from build123d import *

# Parameters (mm, degrees)
F0_W      = 254
F0_H      = 203.2
F1_DEPTH  = 3.175
F3_DEPTH  = 25.4
F4_W      = 76.708
F4_H      = 76.708
F5_DEPTH  = 25.4
F6_R      = 38.354
F7_DEPTH  = 25.4
F9_DEPTH  = 25.4
F10_R     = 19.0754
F11_DEPTH = 25.4
F12_W     = 38.608
F12_H     = 38.608
F13_DEPTH = 25.4


with BuildPart() as f1:
    # F0 (on Top) → F1 (new body)
    with BuildSketch(Plane.XY):
        Rectangle(F0_W, F0_H)
    extrude(amount=F1_DEPTH)

    # F2 (on face) → F3 (cut)
    with BuildSketch(Plane(origin=(0, 0, 0), x_dir=(1, 0, 0), z_dir=(0, 0, -1))):
        Polygon((-69.596, 82.55), (-107.95, 5.842), (-31.242, 5.842), align=None)
    extrude(amount=-F3_DEPTH, mode=Mode.SUBTRACT)

    # F4 (on face) → F5 (cut)
    with BuildSketch(Plane(origin=(0, 0, 0), x_dir=(1, 0, 0), z_dir=(0, 0, -1))):
        with Locations((12.446, -44.196)):
            Rectangle(F4_W, F4_H)
    extrude(amount=-F5_DEPTH, mode=Mode.SUBTRACT)

    # F6 (on face) → F7 (cut)
    with BuildSketch(Plane(origin=(0, 0, 0), x_dir=(1, 0, 0), z_dir=(0, 0, -1))):
        with Locations((68.326, 45.466)):
            Circle(F6_R)
    extrude(amount=-F7_DEPTH, mode=Mode.SUBTRACT)

    # F8 (on face) → F9 (cut)
    with BuildSketch(Plane(origin=(0, 0, 0), x_dir=(1, 0, 0), z_dir=(0, 0, -1))):
        Polygon((94.512347, -42.973466), (75.208347, -81.581466), (113.816347, -81.581466), align=None)
    extrude(amount=-F9_DEPTH, mode=Mode.SUBTRACT)

    # F10 (on face) → F11 (cut)
    with BuildSketch(Plane(origin=(0, 0, 0), x_dir=(1, 0, 0), z_dir=(0, 0, -1))):
        with Locations((-76.1746, -44.4246)):
            Circle(F10_R)
    extrude(amount=-F11_DEPTH, mode=Mode.SUBTRACT)

    # F12 (on face) → F13 (cut)
    with BuildSketch(Plane(origin=(0, 0, 0), x_dir=(1, 0, 0), z_dir=(0, 0, -1))):
        with Locations((-10.528486, 59.436)):
            Rectangle(F12_W, F12_H)
    extrude(amount=-F13_DEPTH, mode=Mode.SUBTRACT)


solid = f1.part
Work out the finished part from the listing and answer in its coordinate system (mm). A direction names the side the tool comes from. Give positions to 0.01 mm unless a question says otherwise; leave off trailing zeros. Loops run counter-clockwise (first coordinate to the right, second up) from the corner with the lowest first, then second, coordinate; pieces in that order, holes last. Notation, with made-up numbers: (-39, 69) -> (-11, 69) arc R14 ccw to (-11, 83) -> close; hole circle Ø2 at (-38.75, 15.25). An arc over 180 degrees is marked (long way). Use a Markdown table: item, result. Add a question column.
1) For a pull along Y with two mould halves and no side action, classify faces 1 (the flat face through (-50.15, -43.66, 1.57)), 2 (the flat face through (-2, 1, 3.175)), 3 (the cylindrical face through (-78.66, 25.51, 1.57)) as +Y half, -Y half, draft (parallel to the pull), parting line (faces both ways), or undercut.
2) Consider line 1 along Y through (x, z) = (-7.5, 2.65); line 2 along X through (y, z) = (-24, 0.75); line 3 along Y through (x, z) = (24, 0.6). Determine where each line is inside the solid, lowest interval first.
3) The part is cut by section C-C, the plane y = -65.5. Determine the outline of the cut face in (x, z) (3 decimals), plus the area to 3 significant figures.
4) Which of the six approach directions +Z, -Z, +X, -X, +Y, -Y give full straight-line access (tool end or side, diameter ignored) to faces 4 (the flat face through (-2, 1, 0)), 5 (the flat face through (85, 62, 2))?
5) This flat-tipped pin is pushed along its axis until it touches: P1, Ø5, axis at x = 47, y = 64.5, coming from the +Z side (3 decimals). Where does it stop, or does it pass through?
6) The part is cut by section B-B, the plane x = -1. Determine the outline of the cut face in (y, z) (3 decimals).
7) The part is cut by section D-D, the plane z = 2.1. Determine the outline of the cut face in (x, y), plus the area to 3 significant figures.
8) The part is cut by section A-A, the plane x = 26.5. Determine the outline of the cut face in (y, z) (3 decimals), plus the area to 3 significant figures.
Reported:
| question | item | result |
|---|---|---|
| 1 | face 1 | undercut |
| 1 | face 2 | draft |
| 1 | face 3 | undercut |
| 2 | line 1 | y = -101.6 to -78.74, -40.13 to 5.84, 82.55 to 101.6 |
| 2 | line 2 | x = -127 to -98.87, -40.32 to 36.54, 100.11 to 127 |
| 2 | line 3 | y = -101.6 to 5.84, 82.55 to 101.6 |
| 3 | outline | (-127, 0) -> (-78.121, 0) -> (-78.121, 3.175) -> (-127, 3.175) -> close; (-61.071, 0) -> (-29.832, 0) -> (-29.832, 3.175) -> (-61.071, 3.175) -> close; (8.776, 0) -> (35.62, 0) -> (35.62, 3.175) -> (8.776, 3.175) -> close; (101.032, 0) -> (127, 0) -> (127, 3.175) -> (101.032, 3.175) -> close |
| 3 | area | 422 mm^2 |
| 4 | face 4 | -Z, +X, -X, +Y, -Y |
| 4 | face 5 | +Z, -Z |
| 5 | P1 | passes through |
| 6 | outline | (-101.6, 0) -> (-78.74, 0) -> (-78.74, 3.175) -> (-101.6, 3.175) -> close; (-40.132, 0) -> (5.842, 0) -> (5.842, 3.175) -> (-40.132, 3.175) -> close; (82.55, 0) -> (101.6, 0) -> (101.6, 3.175) -> (82.55, 3.175) -> close |
| 7 | outline | (-127, -101.6) -> (127, -101.6) -> (127, 101.6) -> (-127, 101.6) -> close; hole (-107.95, -5.84) -> (-69.6, -82.55) -> (-31.24, -5.84) -> close; hole circle Ø38.15 at (-76.17, 44.42); hole (-29.83, -78.74) -> (8.78, -78.74) -> (8.78, -40.13) -> (-29.83, -40.13) -> close; hole (-25.91, 5.84) -> (50.8, 5.84) -> (50.8, 82.55) -> (-25.91, 82.55) -> close; hole circle Ø76.71 at (68.33, -45.47); hole (75.21, 81.58) -> (94.51, 42.97) -> (113.82, 81.58) -> close |
| 7 | area | 34,800 mm^2 |
| 8 | outline | (-101.6, 0) -> (5.842, 0) -> (5.842, 3.175) -> (-101.6, 3.175) -> close; (82.55, 0) -> (101.6, 0) -> (101.6, 3.175) -> (82.55, 3.175) -> close |
| 8 | area | 402 mm^2 |
